Read the model definition and answer for the solid it produces. Units are mm, in the model's axes. Face numbers are marked on the shaded views. A direction names the side the tool comes from. Round coordinates to 2 decimals unless told otherwise and drop trailing zeros. Write each loop counter-clockwise with the first axis right and the second up, starting at its lowest first coordinate (ties: lowest second). Pieces come first, ordered by that corner, then holes. Notation, with made-up numbers: M 13,10.5 L 25,10.5 A15 cw 25,26.5 Z; hole C 60.25,52.5 d1. An arc over 180 degrees is marked long. Use one line per item in the form item = value. Start each with the question number.
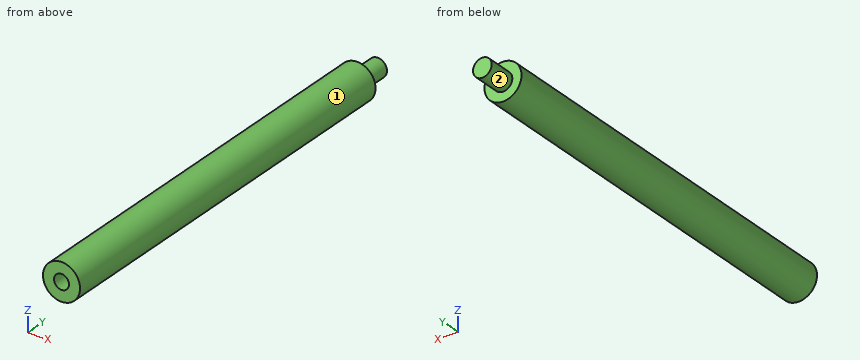
```python
from build123d import *

# Parameters (mm, degrees)
SKETCH2_R                 = 1.984375
BOSS_EXTRUDE1_DEPTH       = 43.6372
SKETCH3_R                 = 1
BOSS_EXTRUDE2_DEPTH       = 3.048
M2X0_4_TAPPED_HOLE1_D     = 1.6
M2X0_4_TAPPED_HOLE1_DEPTH = 5.207
M2X0_4_TAPPED_HOLE1_TIP   = 0.480688495


with BuildPart() as part:
    # Sketch2 → Boss-Extrude1 (new body)
    with BuildSketch(Plane(origin=(0, 0, 0), x_dir=(1, 0, 0), z_dir=(0, 1, 0))):
        Circle(SKETCH2_R)
    extrude(amount=BOSS_EXTRUDE1_DEPTH)

    # Sketch3 → Boss-Extrude2 (add)
    with BuildSketch(Plane(origin=(0, 43.6372, 0), x_dir=(1, 0, 0), z_dir=(0, 1, 0))):
        Circle(SKETCH3_R)
    extrude(amount=BOSS_EXTRUDE2_DEPTH)

    # M2x0.4 Tapped Hole1
    with Locations(Plane(origin=(0, 0, 0), x_dir=(-1, 0, 0), z_dir=(0, -1, 0))):
        with Locations((0, 0)):
            Hole(M2X0_4_TAPPED_HOLE1_D / 2, depth=M2X0_4_TAPPED_HOLE1_DEPTH)
            with Locations((0, 0, -(M2X0_4_TAPPED_HOLE1_DEPTH + M2X0_4_TAPPED_HOLE1_TIP / 2))):  # 118° drill point
                Cone(0, M2X0_4_TAPPED_HOLE1_D / 2, M2X0_4_TAPPED_HOLE1_TIP, mode=Mode.SUBTRACT)


solid = part.part
```
Q1. This flat-tipped pin is pushed along its axis until it touches: pin 1 Ø1.4 at (x, z) = (0, 0) entering from -Y. Where does it stop, or does it pass through?
Q2. Straight lines are drawn through the part: line 1 (Z direction, x = 0, y = 2.8); line 2 (Y direction, x = 0.45, z = 1.6); line 3 (Z direction, x = -0.55, y = 5). For each, find the intervals that lie inside material, in ascending order. Write a range as [from, to].
Q3. Find section A-A on y = 16. Write down the section's boundary in (x, z).
Q4. A tool of negligible diameter and unlimited length cuts with its end or side. For the marked faces 1 and 2, from which of +Z, -Z, +X, -X, +Y, -Y can it reach the whole face along a straight path? Write none if from no direction.
Q5. Find section B-B on x = 1.45. Write down the section's boundary in (y, z), and give its area (3 significant figures).
Response:
q1.pin_1 = 5.27
q2.line_1 = [-1.98, -0.8], [0.8, 1.98]
q2.line_2 = [0, 43.64]
q2.line_3 = [-1.91, -0.58], [0.58, 1.91]
q3.outline = C 0,0 d3.97
q4.face_1 = +Y, -Y
q4.face_2 = +Y
q5.outline = M 0,-1.35 L 43.64,-1.35 L 43.64,1.35 L 0,1.35 Z
q5.area = 118 mm²
